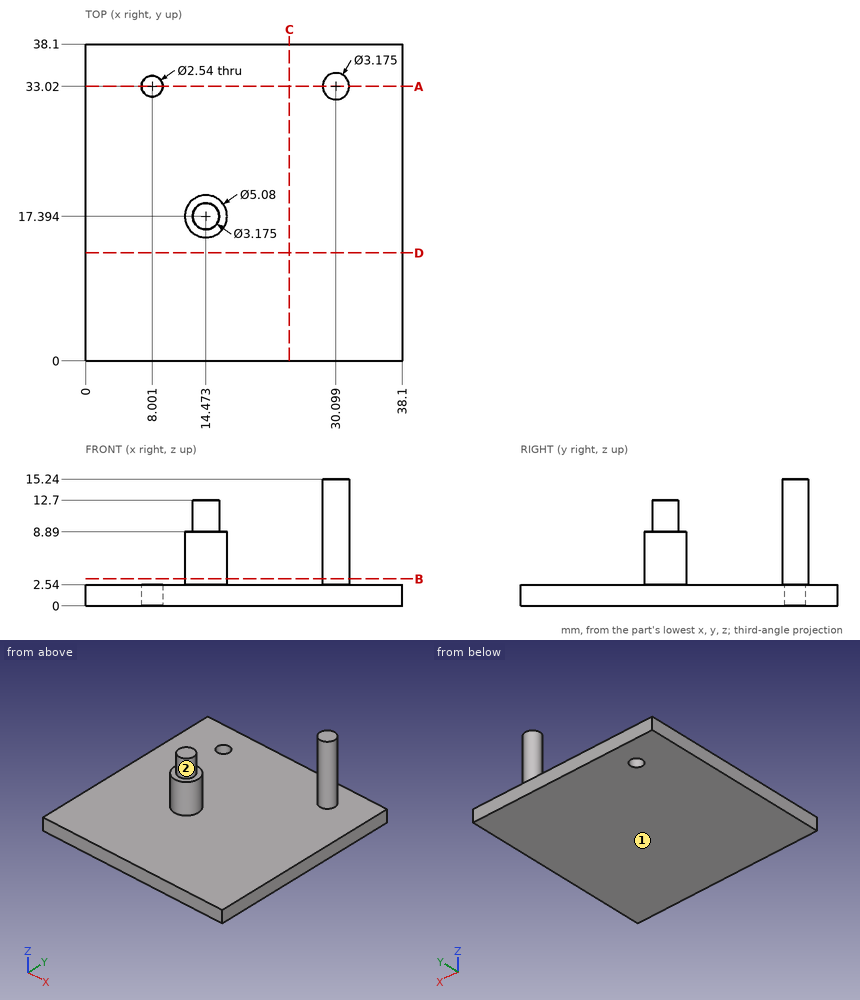
Here's the drawing with two shaded views (mm, measured from the low corner). I have some questions. A direction names the side the tool comes from. Round coordinates to 2 decimals unless told otherwise and drop trailing zeros. Loops run counter-clockwise (first coordinate to the right, second up) from the corner with the lowest first, then second, coordinate; pieces in that order, holes last. Notation, with made-up numbers: (74, 17) - (131, 17) arc R17 cw to (131, 25) - close; hole circle Ø3 at (57.25, 24.5). An arc over 180 degrees is marked (long way). Use CSV: the item, a comma, the result in double quotes. Start each with the question number.
1) If we section it at C-C on x = 24.5: Write out the boundary of the cut face in (y, z).
2) Please list where these lines run through material, in increasing order: probe 1 along X at (y, z) = (33.02, 1.5); probe 2 along Z at (x, y) = (11.5, 22); probe 3 along X at (y, z) = (17.5, 7) (1 decimal). Write a range as [from, to].
3) For pin 1 Ø11.5 at (x, y) = (26.5, 11) entering from +Z; pin 2 Ø1 at (x, y) = (15.5, 18) entering from +Z; pin 3 Ø8 at (x, y) = (18.5, 26) entering from -Z; pin 4 Ø6 at (x, z) = (18, 9) entering from +Y, each with a flat end and sliding along its axis, tell me the tip position at first contact or that it passes through.
4) If we section it at B-B on z = 3.25: Write out the boundary of the cut face in (x, y) (1 decimal).
5) If we section it at A-A on y = 33.02: Write out the boundary of the cut face in (x, z).
6) For the marked faces 1 and 2, which set-ups out of +Z, -Z, +X, -X, +Y, -Y let a thin tool reach every point of the face, with its end or its side?
Geometry results:
1,outline,"(0, 0) - (38.1, 0) - (38.1, 2.54) - (0, 2.54) - close"
2,probe 1,"x = [0, 6.73], [9.27, 38.1]"
2,probe 2,"z = [0, 2.54]"
2,probe 3,"x = [11.9, 17]"
3,pin 1,"stops at z = 2.54"
3,pin 2,"stops at z = 12.7"
3,pin 3,"stops at z = 0"
3,pin 4,"stops at y = 19.88"
4,outline,"circle Ø5.1 at (14.5, 17.4); circle Ø3.2 at (30.1, 33)"
5,outline,"(0, 0) - (6.73, 0) - (6.73, 2.54) - (0, 2.54) - close; (9.27, 0) - (38.1, 0) - (38.1, 2.54) - (31.69, 2.54) - (31.69, 15.24) - (28.51, 15.24) - (28.51, 2.54) - (9.27, 2.54) - close"
6,face 1,"-Z, +X, -X, +Y, -Y"
6,face 2,"+Z"
